Geometry check sheet. Reference: the model listing, model coordinates, mm. Face numbers are marked on the shaded views. A direction names the side the tool comes from. Give positions to 0.01 mm unless a question says otherwise; leave off trailing zeros. Loops run counter-clockwise (first coordinate to the right, second up) from the corner with the lowest first, then second, coordinate; pieces in that order, holes last. Notation, with made-up numbers: (-16, 49.25) -> (15, 49.25) arc R15 cw to (15, 60.25) -> close; hole circle Ø8 at (41, 57.25). An arc over 180 degrees is marked (long way). Write item = value, one per line.
```python
from build123d import *

# Parameters (mm, degrees)
SKETCH_1_R          = 1.5
EXTRUDE_2_DEPTH     = 3
EXTRUDE_3_DEPTH     = 4
SKETCH_3_R          = 1.6
CUT_EXTRUDE_1_DEPTH = 5
FILLET_1_R          = 5
FILLET_2_R          = 1
FILLET_3_R          = 1


with BuildPart() as part:
    # 草图1 → 凸台-拉伸2 (new body)
    with BuildSketch(Plane.XY):
        with BuildLine():
            Line((6, -14), (14, -14))
            Line((14, -14), (14, 14))
            Line((14, 14), (0.634428877, 14))
            ThreePointArc((0.634428877, 14), (0, 5.95), (-0.634428877, 14))
            Line((-0.634428877, 14), (-14, 14))
            Line((-14, 14), (-14, -14))
            Line((-14, -14), (-6, -14))
            Line((-6, -14), (-6, 0))
            Line((-6, 0), (6, 0))
            Line((6, 0), (6, -14))
        make_face()
        with Locations((-10, 10)):
            Circle(SKETCH_1_R, mode=Mode.SUBTRACT)
        with Locations((10, 10)):
            Circle(SKETCH_1_R, mode=Mode.SUBTRACT)
        with Locations((10, -10)):
            Circle(SKETCH_1_R, mode=Mode.SUBTRACT)
        with Locations((-10, -10)):
            Circle(SKETCH_1_R, mode=Mode.SUBTRACT)
    extrude(amount=EXTRUDE_2_DEPTH)

    # 草图2 → 凸台-拉伸3 (add)
    with BuildSketch(Plane.XZ.offset(14)):
        Polygon((6, 3), (14, 3), (14, -12), (-14, -12), (-14, 3), (-6, 3), (-6, -2), (6, -2), align=None)
    extrude(amount=EXTRUDE_3_DEPTH)

    # 草图3 → 切除-拉伸1 (cut)
    with BuildSketch(Plane(origin=(0, -14, 0), x_dir=(1, 0, 0), z_dir=(0, 1, 0))):
        with Locations(Location((-7, 9, 0), (0, 0, 270))):
            Circle(SKETCH_3_R)
        with Locations(Location((7, 9, 0), (0, 0, 90))):
            Circle(SKETCH_3_R)
    extrude(amount=-CUT_EXTRUDE_1_DEPTH, mode=Mode.SUBTRACT)

    # 圆角1
    fillet_1_edges = [part.edges().sort_by_distance(p)[0] for p in [
        (-14, 14, 1.5),
        (-0.634428877, 14, 1.5),
        (0.634428877, 14, 1.5),
        (14, 14, 1.5),
        (-14, -16, -12),
        (14, -16, -12),
    ]]
    fillet(fillet_1_edges, radius=FILLET_1_R)

    # 圆角2
    fillet_2_edges = [part.edges().sort_by_distance(p)[0] for p in [
        (0, 0, 0),
        (-6, -7, 0),
        (-10, -14, 0),
        (14, -2.5, 0),
        (-14, -14, -3.5),
        (6, -14, -1),
        (0, -14, -2),
        (-6, -14, -1),
        (-8.997290851, 14, 0),
        (-14, -2.5, 0),
        (0, 5.95, 0),
        (8.997290851, 14, 0),
        (12.535533906, 12.535533906, 0),
        (-12.535533906, 12.535533906, 0),
        (5.660097555, 12.725750323, 0),
        (-5.660097555, 12.725750323, 0),
        (10, -14, 0),
        (14, -14, -3.5),
        (0, -14, -12),
        (6, -7, 0),
        (12.535533906, -14, -10.535533906),
        (-12.535533906, -14, -10.535533906),
    ]]
    fillet(fillet_2_edges, radius=FILLET_2_R)

    # 圆角3
    fillet_3_edges = [part.edges().sort_by_distance(p)[0] for p in [
        (14, -4.5, 3),
        (-8.997290851, 14, 3),
        (0, 5.95, 3),
        (8.997290851, 14, 3),
        (-14, -4.5, 3),
        (12.535533906, 12.535533906, 3),
        (-12.535533906, 12.535533906, 3),
        (5.660097555, 12.725750323, 3),
        (-5.660097555, 12.725750323, 3),
    ]]
    fillet(fillet_3_edges, radius=FILLET_3_R)


solid = part.part
```
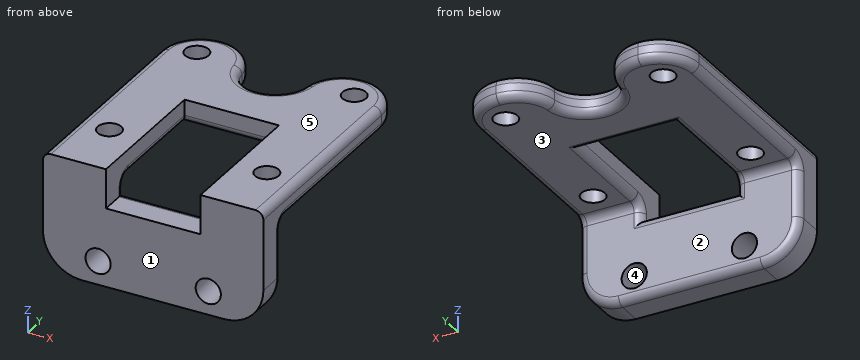
Item 1: Tool access check on the marked faces 1 and 2. Record the directions out of +Z, -Z, +X, -X, +Y, -Y that give a thin tool (end or side, any length) a straight path to the whole face; none if there is none.
Answer:
face_1 = +Z, -Z, +X, -X, -Y
face_2 = -Z, +X, -X, +Y
Item 2: Section check A-A, the plane y = -5. Record the cut outline in (x, z).
Answer:
outline = (-14, 1) arc R1 ccw to (-13, 0) -> (-7, 0) arc R1 ccw to (-6, 1) -> (-6, 3) -> (-13, 3) arc R1 ccw to (-14, 2) -> close; (6, 1) arc R1 ccw to (7, 0) -> (13, 0) arc R1 ccw to (14, 1) -> (14, 2) arc R1 ccw to (13, 3) -> (6, 3) -> close
Item 3: Section check C-C, the plane x = -10. Give the number of separate pieces and of enclosed holes in the cut face, plus the area to 3 significant figures.
Answer:
separate_pieces = 3
enclosed_holes = 0
area = 125 mm^2
Item 4: Draft check along Z on the marked faces 3, 4 and 5. Enter one of: +Z half, -Z half, draft (parallel to the pull), parting line (faces both ways), or undercut.
Answer:
face_3 = -Z half
face_4 = undercut
face_5 = +Z half
Item 5: Thickness scan on L1, parallel to X at y = -15.3, z = -9; L2, parallel to Z at x = 4, y = -16.5; L3, parallel to Y at x = 7.75, z = -1.5. Record the ranges inside material, lowest first. Write a range as [from, to].
Answer:
L1 = [-13.58, -8.6], [-5.4, 5.4], [8.6, 13.58]
L2 = [-12, -2]
L3 = [-18, -14]
Item 6: Gauge pin test, flat ends, axial feed: pin 1 (3 mm diameter, centred on x = 4, z = -6.5, fed in from +Y); pin 2 (5 mm diameter, centred on x = 10, y = 10, fed in from -Z); pin 3 (5 mm diameter, centred on y = -3, z = -2, fed in from +X). Record the tip position at first contact, or that the pin passes through.
Answer:
pin_1 = -14
pin_2 = 0
pin_3 = 13.87
Item 7: Section check B-B, the plane y = -10. Record the cut outline in (x, z).
Answer:
outline = (-14, 1) arc R1 ccw to (-13, 0) -> (-11.5, 0) -> (-11.5, 3) -> (-13, 3) arc R1 ccw to (-14, 2) -> close; (-8.5, 0) -> (-7, 0) arc R1 ccw to (-6, 1) -> (-6, 3) -> (-8.5, 3) -> close; (6, 1) arc R1 ccw to (7, 0) -> (8.5, 0) -> (8.5, 3) -> (6, 3) -> close; (11.5, 0) -> (13, 0) arc R1 ccw to (14, 1) -> (14, 2) arc R1 ccw to (13, 3) -> (11.5, 3) -> close
